CAD build for the part. Positions are in the model's coordinates, mm. Face numbers are marked on the shaded views. A direction names the side the tool comes from. Round coordinates to 2 decimals unless told otherwise and drop trailing zeros. Write each loop counter-clockwise with the first axis right and the second up, starting at its lowest first coordinate (ties: lowest second). Pieces come first, ordered by that corner, then holes. Notation, with made-up numbers: (83.25, 3) -> (134.25, 3) arc R17 cw to (134.25, 36) -> close; hole circle Ø11 at (83.25, 80.25). An arc over 180 degrees is marked (long way). Put each result on its own line as item: value. Start each with the question number.
1. Saw through at C-C on z = 18.25. List the corners of the cut face in (x, y).
2. Saw through at A-A on x = 7.5. List the corners of the cut face in (y, z), and give its area (3 significant figures).
3. 3-axis set-ups, long thin cutter, end or side, ignore diameter. For the marked faces 4, 5 and 6: which of +Z, -Z, +X, -X, +Y, -Y reach the whole face in a straight line?
4. Flat gauge pins, fed straight in: P1, Ø8, axis at x = 18.5, z = 16, coming from the +Y side; P2, Ø0.8, axis at x = 0, z = 20.5, coming from the -Y side; P3, Ø10, axis at y = -4, z = 16, coming from the +X side. Where does each tip first touch, or does it go through?
5. Drill centre lines: line 1 (Y direction, x = 0, z = 16.5); line 2 (X direction, y = -0.5, z = 8.75); line 3 (Y direction, x = 6.5, z = 7.5). Where is each one in solid material? Low to high. Write a range as from..to.
6. Saw through at B-B on y = -8. List the corners of the cut face in (x, z).
7. Pull direction Z, two halves, no side cores. Call the marked faces 1, 2 and 3: pulls with the +Z half, pulls with the -Z half, needs draft (parallel to the pull), parting line crosses it, or undercut.
8. Saw through at D-D on x = -17. List the corners of the cut face in (y, z), and give its area (3 significant figures).
from build123d import *

# Parameters (mm, degrees)
F4_START = 14
F4_DEPTH = 16
F5_START = 20
F5_DEPTH = 1


with BuildPart() as f3:
    # F0 (on Front) → F3 (revolve)
    with BuildSketch(Plane.XZ):
        Polygon((0, 7), (0, 0), (22.2, 0), (22.2, 21), (15.1, 21), (15.1, 7), align=None)
    revolve(axis=Axis((0, 0, 3.5), (0, 0, -1)))

    # F1 (on Right) → F4 (cut)
    with BuildSketch(Plane.YZ.offset(F4_START)):
        with BuildLine():
            Line((4.5, 21.0452601314), (0, 21.0452601314))
            Line((0, 21.0452601314), (-4.5, 21.0452601314))
            Line((-4.5, 21.0452601314), (-4.5, 11.0452601314))
            ThreePointArc((-4.5, 11.0452601314), (0, 6.5452601314), (4.5, 11.0452601314))
            Line((4.5, 11.0452601314), (4.5, 21.0452601314))
        make_face()
    extrude(amount=F4_DEPTH, mode=Mode.SUBTRACT)

    # F2 (on Top) → F5 (cut)
    with BuildSketch(Plane.XY.offset(F5_START)):
        Polygon((0.5, -19.3967004567), (0, -19.3967004567), (-0.5, -19.3967004567), (-0.5, -22.3967004567), (0.5, -22.3967004567), align=None)
        Polygon((0.4999070801, 22.4221755646), (-9.29199e-05, 22.4221755646), (-0.5000929199, 22.4221755646), (-0.5000929199, 19.4221755646), (0.4999070801, 19.4221755646), align=None)
        Polygon((22.3929286003, -0.5), (22.3929286003, 0), (22.3929286003, 0.5), (19.3929286003, 0.5), (19.3929286003, -0.5), align=None)
        Polygon((-19.404573366, -0.5), (-19.404573366, 0), (-19.404573366, 0.5), (-22.404573366, 0.5), (-22.404573366, -0.5), align=None)
    extrude(amount=F5_DEPTH, mode=Mode.SUBTRACT)


solid = f3.part
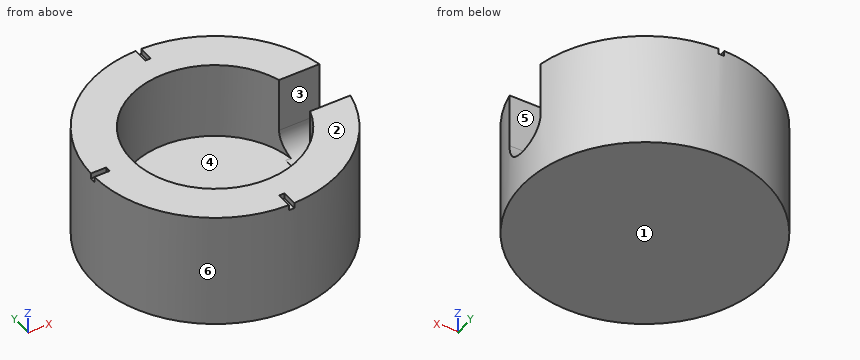
Return value:
1. outline: (14.41, -4.5) arc R15.1 cw (long way) to (14.41, 4.5) -> (21.74, 4.5) arc R22.2 ccw (long way) to (21.74, -4.5) -> close
2. outline: (-20.89, 0) -> (20.89, 0) -> (20.89, 21) -> (13.11, 21) -> (13.11, 7) -> (-13.11, 7) -> (-13.11, 21) -> (-20.89, 21) -> close
2. area: 511 mm^2
3. face 4: +Z
3. face 5: +Z, +X
3. face 6: +Z, -Z
4. P1: stops at y = 16.81
4. P2: stops at y = -19.4
4. P3: stops at x = 21.74
5. line 1: y = -22.2..-15.1, 15.1..22.2
5. line 2: x = -22.19..-15.09
5. line 3: y = -21.23..-13.63, 13.63..21.23
6. outline: (-20.71, 0) -> (20.71, 0) -> (20.71, 21) -> (12.81, 21) -> (12.81, 7) -> (-12.81, 7) -> (-12.81, 21) -> (-20.71, 21) -> close
7. face 1: pulls with the -Z half
7. face 2: pulls with the +Z half
7. face 3: needs draft
8. outline: (-14.28, 0) -> (14.28, 0) -> (14.28, 21) -> (-14.28, 21) -> close
8. area: 600 mm^2
